Here's how the part is built. I have some questions about the finished solid (model axes, mm). A direction names the side the tool comes from. Coordinates: 2 decimals unless noted, no trailing zeros. Write each loop counter-clockwise with the first axis right and the second up, starting at its lowest first coordinate (ties: lowest second). Pieces come first, ordered by that corner, then holes. Notation, with made-up numbers: (17.5, 43.25) -> (56.5, 43.25) arc R35 ccw to (56.5, 78.25) -> close; hole circle Ø5 at (70.5, -32). An arc over 180 degrees is marked (long way). Put each result on its own line as item: value. Start each with the question number.
Item 1: I need wall thicknesses on line 1 (Z direction, x = 2.5, y = -21); line 2 (Z direction, x = 2, y = -10); line 3 (X direction, y = -19, z = 24.5). Which ranges of each line are inside material? Lowest first, please. Write a range as [from, to].
Item 2: On a 3-axis mill with a long thin cutter (end or side, diameter ignored), from which of +Z, -Z, +X, -X, +Y, -Y can I reach the whole of each face in a straight line? I mean faces 5 (the face through (3, -15, 22.949)), 6 (the face through (31.583, -15, 0)), 7 (the face through (-20, -15, 21)), 8 (the face through (-7, 0, 12)), 9 (the face through (41.358, -14.79, 20.349)). Say none if no direction works.
Item 3: I want a section at D-D, the plane x = -29.5. List the corners of the cut face in (y, z) for me, then the cut area to 3 significant figures.
Item 4: If we mould it in two halves opening along X, with no side actions, what happens to faces 1 (the face through (-27, -15, 12.949)), 2 (the face through (32.393, -14.79, 20.486)), 3 (the face through (26.69, -14.79, 28.703)), 4 (the face through (5, -15, 28))? For each: released by +X, released by -X, zero draft, split by the parting line, or undercut.
Item 5: I want a section at C-C, the plane z = -1. List the corners of the cut face in (x, y) for me.
Item 6: For pin 1 (3 mm diameter, centred on y = -17, z = 26.5, fed in from -X); pin 2 (3 mm diameter, centred on x = 9.5, y = -21.5, fed in from +Z); pin 3 (12 mm diameter, centred on x = 2.5, z = 7.95, fed in from +Y); pin 4 (1 mm diameter, centred on y = -23.5, z = 11, fed in from -X), each with a flat end and sliding along its axis, tell me the tip position at first contact or that it passes through.
Item 7: I want a section at B-B, the plane x = 2.5. List the corners of the cut face in (y, z) for me.
Item 8: I want a section at A-A, the plane y = -18.5. List the corners of the cut face in (x, z) for me, then the cut area to 3 significant figures.
from build123d import *

# Parameters (mm, degrees)
F0_R     = 10
F1_DEPTH = 30


with BuildPart() as f1:
    # F0 (on Front) → F1 (new body)
    with BuildSketch(Plane.XZ):
        with BuildLine():
            Line((27.499998, 41.240266), (15, 32.948701))
            Line((15, 32.948701), (5, 32.948701))
            Line((5, 32.948701), (5, 22.948701))
            Line((5, 22.948701), (0, 22.948701))
            Line((0, 22.948701), (0, 32.948701))
            Line((0, 32.948701), (-15, 32.948701))
            ThreePointArc((-15, 32.948701), (-18.535534, 31.484235), (-20, 27.948701))
            Line((-20, 27.948701), (-20, 12.948702))
            Line((-20, 12.948702), (-33.41687, 12.948702))
            ThreePointArc((-33.41687, 12.948702), (-36.952404, 11.484236), (-38.41687, 7.948702))
            Line((-38.41687, 7.948702), (-38.41687, -2.051296))
            ThreePointArc((-38.41687, -2.051296), (-36.952404, -5.58683), (-33.41687, -7.051296))
            Line((-33.41687, -7.051296), (31.58313, -7.051296))
            Line((31.58313, -7.051296), (31.58313, 7.948704))
            Line((31.58313, 7.948704), (44.083128, 16.240268))
            Line((44.083128, 16.240268), (38.555418, 24.5736))
            Line((38.555418, 24.5736), (26.05542, 16.282036))
            Line((26.05542, 16.282036), (23.291564, 20.448704))
            Line((23.291564, 20.448704), (20.52771, 24.615369))
            Line((20.52771, 24.615369), (33.027708, 32.906933))
            Line((33.027708, 32.906933), (27.499998, 41.240266))
        make_face()
        with Locations((2.5, 7.948704)):
            Circle(F0_R, mode=Mode.SUBTRACT)
    extrude(amount=F1_DEPTH)


solid = f1.part
Calculated:
1. line 1: z = [-7.05, -2.05], [17.95, 22.95]
1. line 2: z = [-7.05, -2.04], [17.94, 22.95]
1. line 3: x = [-20, 0], [5, 20.6], [38.44, 38.6]
2. face 5: +Z, +Y, -Y
2. face 6: -Z, +X, +Y, -Y
2. face 7: +Z, -X, +Y, -Y
2. face 8: +Z, -Z, +X, -X, +Y
2. face 9: +Z, +X, +Y, -Y
3. outline: (-30, -7.05) -> (0, -7.05) -> (0, 12.95) -> (-30, 12.95) -> close
3. area: 600 mm2
4. face 1: zero draft
4. face 2: undercut
4. face 3: released by +X
4. face 4: undercut
5. outline: (-38.42, -30) -> (-1.96, -30) -> (-1.96, 0) -> (-38.42, 0) -> close; (6.96, -30) -> (31.58, -30) -> (31.58, 0) -> (6.96, 0) -> close
6. pin 1: stops at x = -20
6. pin 2: stops at z = 32.95
6. pin 3: passes through
6. pin 4: stops at x = -37.72
7. outline: (-30, -7.05) -> (0, -7.05) -> (0, -2.05) -> (-30, -2.05) -> close; (-30, 17.95) -> (0, 17.95) -> (0, 22.95) -> (-30, 22.95) -> close
8. outline: (-38.42, -2.05) arc R5 ccw to (-33.42, -7.05) -> (31.58, -7.05) -> (31.58, 7.95) -> (44.08, 16.24) -> (38.56, 24.57) -> (26.06, 16.28) -> (20.53, 24.62) -> (33.03, 32.91) -> (27.5, 41.24) -> (15, 32.95) -> (5, 32.95) -> (5, 22.95) -> (0, 22.95) -> (0, 32.95) -> (-15, 32.95) arc R5 ccw to (-20, 27.95) -> (-20, 12.95) -> (-33.42, 12.95) arc R5 ccw to (-38.42, 7.95) -> close; hole circle Ø20 at (2.5, 7.95)
8. area: 2,140 mm2
